Part model, mm, in its own coordinate system. Round coordinates to 2 decimals unless told otherwise and drop trailing zeros. Write each loop counter-clockwise with the first axis right and the second up, starting at its lowest first coordinate (ties: lowest second). Pieces come first, ordered by that corner, then holes. Notation, with made-up numbers: M -1.5,2 L 33.5,2 A3 cw 33.5,6 Z; hole C 60,61.5 d11. An arc over 180 degrees is marked long. Answer as a JSON object with one key per item and string values. Group by question number.
1. Drop a flat-ended pin along its axis: pin 1 (2.5 mm diameter, centred on x = -1.58, z = 48.26, fed in from -Y). Give the stop position or say it passes through.
2. Band-saw the part on D-D, the plane x = -22.5. Write the cut outline in (y, z), plus the area to 3 significant figures.
3. Band-saw the part on B-B, the plane z = 0. Write the cut outline in (x, y).
4. Band-saw the part on A-A, the plane x = 37.5. Write the cut outline in (y, z).
5. Band-saw the part on C-C, the plane z = 22.5. Write the cut outline in (x, y).
6. Drill centre lines: line 1 (Z direction, x = 34.5, y = 2.45); line 2 (Z direction, x = 24, y = 4.4); line 3 (Z direction, x = 4.5, y = 2.3). Where is each one in solid material? Low to high. Write a range as from..to.
7. Two-plate mould, pull along Z, no slides. Class faces 1 (the face through (36.3, 2.5, 6.1)), 2 (the face through (62.44, 2.46, -2.75)), 3 (the face through (15, 5, 15)): +Z half, -Z half, draft (parallel to the pull), parting line (faces both ways), or undercut.
Autodesk Inventor part; units mm, degrees
ref_plane "YZ Plane" through (0, 0, 0) normal (1, 0, 0) x (0, 1, 0)
ref_plane "XZ Plane" through (0, 0, 0) normal (0, 1, 0) x (-1, 0, 0)
ref_plane "XY Plane" through (0, 0, 0) normal (0, 0, 1) x (1, 0, 0)
sketch "Sketch1" plane through (0, 0, 0) normal (0, 1, 0) x (-1, 0, 0)
  line L0 (0, 0) -> (50, 0) construction
  line L1 (0, 0) -> (50, 0) construction
  line L2 (0, 0) -> (-36, 0)
  circle A0 centre (0, 0) radius 25
  line L3 (-60, -10) -> (-60, 10)
  circle A1 centre (0, 0) radius 61
  circle A2 centre (0, 0) radius 62.5
  point P0 (62.509, -33.0548)
  point P1 (12.6591, 21.558)
  point P2 (24.4148, 5.3777)
  point P3 (24.4148, -5.3777)
  point P4 (-22.9129, 10)
  point P5 (-22.9129, -10)
  point P6 (12.6591, -21.558)
  dimension "d2" = 36
  dimension "d3" = 50
  dimension "d26" = 122
  dimension "d154" = 125
extrude "Extrusion1" add sketch "Sketch1" along normal blind 5 contours A0 | A1 | A2
sketch "Sketch2" plane through (0, 5, 0) normal (0, 1, 0) x (1, 0, 0)
  circle A0 centre (0, 0) radius 20
  dimension "d6" = 40
extrude "Extrusion2" cut sketch "Sketch2" against normal up to next
sketch "Sketch3" plane through (0, 5, 0) normal (0, 1, 0) x (1, 0, 0)
  line L0 (22.1416, 4) -> (20.8701, 4)
  line L1 (22.1416, -4) -> (20.8701, -4)
  line L2 (24.6779, 4) -> (22.1416, 4)
  line L3 (24.6779, -4) -> (22.1416, -4)
  line L4 (-15.5618, -16.2506) -> (-14.5332, -15.5032)
  line L5 (-15.5618, 16.2506) -> (-14.5332, 15.5032)
  line L6 (-20.2641, -9.7784) -> (-19.2354, -9.0311)
  line L7 (-17.6137, -17.7414) -> (-15.5618, -16.2506)
  line L8 (-22.316, -11.2693) -> (-20.2641, -9.7784)
  line L9 (-20.2641, 9.7784) -> (-19.2354, 9.0311)
  line L10 (-17.6137, 17.7414) -> (-15.5618, 16.2506)
  line L11 (-22.316, 11.2693) -> (-20.2641, 9.7784)
  line L12 (-23.5374, 22.0452) -> (-13.679, 22.0452) construction
  arc A0 (-17.6137, -17.7414) -> (24.6779, -4) centre (0, 0) ccw
  arc A1 (24.6779, 4) -> (-17.6137, 17.7414) centre (0, 0) ccw
  arc A2 (-22.316, 11.2693) -> (-22.316, -11.2693) centre (0, 0) ccw
  line L13 (20.8701, 4) -> (15.8701, 4)
  line L14 (15.8701, 4) -> (15.8701, -4)
  line L15 (15.8701, -4) -> (20.8701, -4)
  line L16 (-14.5332, 15.5032) -> (-10.4881, 12.5643)
  line L17 (-10.4881, 12.5643) -> (-15.1903, 6.0922)
  line L18 (-15.1903, 6.0922) -> (-19.2354, 9.0311)
  line L19 (-19.2354, -9.0311) -> (-15.1903, -6.0922)
  line L20 (-15.1903, -6.0922) -> (-10.4881, -12.5643)
  line L21 (-10.4881, -12.5643) -> (-14.5332, -15.5032)
  circle A3 centre (-22.5, 0) radius 1.5
  circle A4 centre (0, 22.5) radius 1.5
  circle A5 centre (18.2029, 13.2252) radius 1.5
  circle A6 centre (18.2029, -13.2252) radius 1.5
  circle A7 centre (0, -22.5) radius 1.5
  circle A8 centre (0, 0) radius 4
  line L22 (0, 0) -> (8, 0)
  line L23 (8, 0) -> (8, 7.5)
  line L24 (8, 0) -> (8, -7.5)
  circle A9 centre (8, -7.5) radius 2.5
  circle A10 centre (8, 7.5) radius 2.5
  point P0 (-23.5374, -22.0452)
  point P1 (-28.2397, -15.5731)
  dimension "d9" = 36
  dimension "d10" = 5
  dimension "d11" = 5
  dimension "d12" = 3
  dimension "d13" = 3
  dimension "d14" = 3
  dimension "d15" = 3
  dimension "d16" = 3
  dimension "d17" = 8
  dimension "d18" = 8
  dimension "d19" = 7.5
  dimension "d20" = 7.5
  dimension "d21" = 5
  dimension "d22" = 5
extrude "Extrusion3" cut sketch "Sketch3" against normal up to next contours A3 | A4 | A5 | A6 | A7
sketch "Sketch5" plane through (0, 5, 0) normal (0, 1, 0) x (1, 0, 0)
  line L0 (0, 0) -> (37.5601, 0) construction
  circle A0 centre (0, 0) radius 25
  line L1 (0, 0) -> (15.7675, -27.31)
  line L2 (0, 0) -> (31.5349, 0) construction
  line L3 (0, 0) -> (19.8269, 34.3411)
  line L4 (0, 0) -> (39.6537, 0) construction
  line L5 (12.5, 21.6506) -> (15, 25.9808)
  line L6 (12.5, -21.6506) -> (15, -25.9808)
  line L7 (15, -25.9808) -> (27.9904, -18.4808)
  line L8 (27.9904, -18.4808) -> (34.9904, -30.6051)
  line L9 (34.9904, -30.6051) -> (22, -38.1051)
  line L10 (22, -38.1051) -> (15, -25.9808)
  line L11 (22, -38.1051) -> (15, -25.9808)
  line L12 (15, -25.9808) -> (2.0096, -33.4808)
  line L13 (2.0096, -33.4808) -> (9.0096, -45.6051)
  line L14 (9.0096, -45.6051) -> (22, -38.1051)
  line L15 (15, 25.9808) -> (2.0096, 33.4808)
  line L16 (2.0096, 33.4808) -> (9.0096, 45.6051)
  line L17 (9.0096, 45.6051) -> (22, 38.1051)
  line L18 (22, 38.1051) -> (15, 25.9808)
  line L19 (22, 38.1051) -> (15, 25.9808)
  line L20 (15, 25.9808) -> (27.9904, 18.4808)
  line L21 (27.9904, 18.4808) -> (34.9904, 30.6051)
  line L22 (34.9904, 30.6051) -> (22, 38.1051)
  dimension "d41" = 50
  dimension "d47" = 60
  dimension "d48" = 60
  dimension "d49" = 5
  dimension "d50" = 5
  dimension "d51" = 15
  dimension "d52" = 14
  dimension "d53" = 15
  dimension "d54" = 15
  dimension "d55" = 14
  dimension "d56" = 15
extrude "Extrusion5" cut sketch "Sketch5" against normal up to next contours L7 L8 L9 L10 L1 | L1 L10 L14 L13 L12 | L15 L16 L17 L18 L3 | L3 L18 L22 L21 L20
sketch "Sketch8" plane through (0, 0, 0) normal (0, -1, 0) x (1, 0, 0)
  line L0 (-37.9479, -22.6265) -> (-41.4746, -17.7724)
  line L1 (-47.9467, -22.4747) -> (-44.42, -27.3288)
  line L2 (-31.2231, -27.6292) -> (-27.6611, -32.4577)
  circle A0 centre (-42.9473, -22.5506) radius 1.5
  circle A1 centre (-26.2405, -27.6816) radius 1.5
  line L3 (-29.7189, 33.9527) -> (-36.191, 38.655)
  line L4 (-39.7177, 33.8009) -> (-33.2456, 29.0986)
  line L5 (-29.4532, 16.4547) -> (-35.9253, 21.157)
  line L6 (41.5, 10) -> (33.5, 10)
  line L7 (33.5, 4) -> (41.5, 4)
  line L8 (44, -10) -> (52, -10)
  circle A2 centre (48, -7) radius 1.5
  circle A3 centre (37.5, 7) radius 1.5
  circle A4 centre (-34.7183, 33.8768) radius 1.5
  circle A5 centre (-34.4526, 16.3788) radius 1.5
  point P0 (0, 0)
  point P1 (0, 0)
  point P2 (-32.9799, 11.6006)
  point P3 (44, -4)
  dimension "d73" = 3
  dimension "d74" = 3
  dimension "d75" = 3
  dimension "d76" = 3
  dimension "d77" = 3
extrude "Extrusion8" cut sketch "Sketch8" against normal blind 5
sketch "Sketch9" plane through (0, 5, 0) normal (0, 1, 0) x (1, 0, 0)
  line L0 (2.0096, -33.4808) -> (27.9904, -18.4808)
  line L1 (9.0096, -45.6051) -> (2.0096, -33.4808)
  line L2 (2.0096, -33.4808) -> (-0.5885, -34.9808)
  line L3 (-0.5885, -34.9808) -> (6.4115, -47.1051)
  line L4 (6.4115, -47.1051) -> (9.0096, -45.6051)
  line L5 (2.0096, 33.4808) -> (9.0096, 45.6051)
  line L6 (2.0096, 33.4808) -> (9.0096, 45.6051)
  line L7 (9.0096, 45.6051) -> (6.4115, 47.1051)
  line L8 (6.4115, 47.1051) -> (-0.5885, 34.9808)
  line L9 (-0.5885, 34.9808) -> (2.0096, 33.4808)
  point P0 (0, 0)
  dimension "d80" = 3
  dimension "d81" = 3
extrude "Extrusion9" cut sketch "Sketch9" against normal blind 10
sketch "Sketch10" plane through (0, 0, 0) normal (0, -1, 0) x (1, 0, 0)
  line L0 (6.4115, 47.1051) -> (-9.1769, 56.1051)
  line L1 (-9.1769, 56.1051) -> (-16.1769, 43.9808)
  line L2 (-16.1769, 43.9808) -> (-0.5885, 34.9808)
  line L3 (-9.1769, 56.1051) -> (-11.1769, 52.641)
  line L4 (-16.1769, 43.9808) -> (-14.1769, 47.4449)
  line L5 (-0.5885, 34.9808) -> (1.4115, 38.4449)
  line L6 (1.4115, 38.4449) -> (-2.0526, 40.4449)
  line L7 (6.4115, 47.1051) -> (4.4115, 43.641)
  line L8 (-0.5885, 34.9808) -> (6.4115, 47.1051)
  line L9 (4.4115, 43.641) -> (0.9474, 45.641)
  line L10 (27.9904, -18.4808) -> (-0.5885, -34.9808)
  line L11 (-16.1769, -43.9808) -> (-9.1769, -56.1051)
  line L12 (6.4115, -47.1051) -> (-0.5885, -34.9808)
  line L13 (-16.1769, -43.9808) -> (-14.1769, -47.4449)
  line L14 (-14.1769, -47.4449) -> (-10.7128, -45.4449)
  line L15 (-9.1769, -56.1051) -> (-11.1769, -52.641)
  line L16 (6.4115, -47.1051) -> (4.4115, -43.641)
  line L17 (-0.5885, -34.9808) -> (6.4115, -47.1051)
  line L18 (-0.5885, -34.9808) -> (1.4115, -38.4449)
  line L19 (6.4115, 47.1051) -> (3.8135, 48.6051)
  line L20 (3.8135, 48.6051) -> (-3.1865, 36.4808)
  line L21 (3.8135, 48.6051) -> (-2.6817, 52.3551)
  line L22 (1.8135, 45.141) -> (-2.0836, 47.391)
  line L23 (-2.0836, 47.391) -> (-5.0836, 42.1949)
  line L24 (-0.5885, -34.9808) -> (1.4115, -38.4449)
  line L25 (6.4115, -47.1051) -> (4.4115, -43.641)
  circle A0 centre (-5.5836, -41.3288) radius 1.5
  circle A1 centre (-1.5836, -48.257) radius 1.5
  line L26 (-2.0836, 47.391) -> (-1.5836, 48.257)
  line L27 (-5.0836, 42.1949) -> (-5.5836, 41.3288)
  circle A2 centre (-1.5836, 48.257) radius 1.5
  circle A3 centre (-5.5836, 41.3288) radius 1.5
  point P0 (0, 0)
  dimension "d85" = 14
  dimension "d86" = 4
  dimension "d88" = 4
  dimension "d92" = 4
  dimension "d93" = 4
  dimension "d94" = 4
  dimension "d95" = 4
  dimension "d98" = 18
  dimension "d99" = 4
  dimension "d101" = 4
  dimension "d103" = 4
  dimension "d129" = 3
  dimension "d130" = 7.5
  dimension "d137" = 4.5
  dimension "d140" = 4
  dimension "d146" = 3
  dimension "d148" = 1
  dimension "d149" = 1
  dimension "d150" = 3
  dimension "d151" = 3
extrude "Extrusion13" cut sketch "Sketch10" against normal blind 10 contours A2 L23 L22 | L22 L23 A2 | A0 | A1 | A3
sketch "Sketch11" plane through (0, 5, 0) normal (0, 1, 0) x (1, 0, 0)
  circle A0 centre (0, 0) radius 30
  circle A1 centre (0, 0) radius 30
  circle A2 centre (0, 0) radius 25
  circle A3 centre (0, 0) radius 25
  line L0 (-25, -3) -> (-29.8496, -3)
  line L1 (-24.8193, -3) -> (-25, -3)
  line L2 (-25, 3) -> (-24.8193, 3)
  line L3 (-29.8496, 3) -> (-24.8193, 3)
  line L4 (24.8193, -3) -> (29.8496, -3)
  line L5 (24.8193, 3) -> (29.8496, 3)
extrude "Extrusion14" cut sketch "Sketch11" against normal blind 5 contours A0 L4 A2 L5 | L3 L2 A2 L1 L0 A0
properties part number "upperBasePart2"
Worked answers:
{
 "1": {"pin 1": "passes through"},
 "2": {"outline": "M 0,-58.31 L 5,-58.31 L 5,-1.5 L 0,-1.5 Z; M 0,1.5 L 5,1.5 L 5,58.31 L 0,58.31 Z", "area": "568 mm^2"},
 "3": {"outline": "M -62.5,0 L -30,0 L -30,5 L -62.5,5 Z; M -25,0 L -24,0 L -24,5 L -25,5 Z; M -21,0 L -20,0 L -20,5 L -21,5 Z; M 20,0 L 25,0 L 25,5 L 20,5 Z; M 30,0 L 62.5,0 L 62.5,5 L 30,5 Z"},
 "4": {"outline": "M 0,-50 L 5,-50 L 5,5.5 L 0,5.5 Z; M 0,8.5 L 5,8.5 L 5,50 L 0,50 Z"},
 "5": {"outline": "M -58.31,0 L -1.5,0 L -1.5,5 L -58.31,5 Z; M 1.5,0 L 21.03,0 L 21.03,5 L 1.5,5 Z; M 30.31,0 L 58.31,0 L 58.31,5 L 30.31,5 Z"},
 "6": {"line 1": "z = -52.12..-30.89, -29.76..29.76, 30.89..52.12", "line 2": "z = -57.71..-36.95, -20.78..20.78, 36.95..57.71", "line 3": "z = -62.34..-43.79, -32.04..-19.49, 19.49..32.04, 43.79..62.34"},
 "7": {"face 1": "undercut", "face 2": "parting line", "face 3": "draft"}
}
